from build123d import *

# Parameters (mm, degrees)
F0_W         = 500
F0_H         = 80
F1_DEPTH     = 25
F3_D         = 40
F3_DEPTH     = 25
F3_TIP       = 12.0172123806
F4_D         = 10
F4_DEPTH     = 25
F4_TIP       = 3.0043030951
F2_W         = 38
F2_H         = 28
F5_DEPTH     = 10
F6_T         = 2.5
F6_T3_DEPTH  = 15
F6_T5_DEPTH  = 33
F6_T7_DEPTH  = 29
F6_T9_DEPTH  = 39
F6_T11_DEPTH = 39
F6_T13_DEPTH = 33
F6_T15_DEPTH = 29


# Not quite as in the source:
# - a shell that OpenCascade refuses in one call is made with other operations: the cavity is built on its own and cut out


with BuildPart() as f1:
    # F0 (on Top) → F1 (new body)
    with BuildSketch(Plane.XY):
        Rectangle(F0_W, F0_H)
    extrude(amount=F1_DEPTH)

    # F3
    with Locations(Plane.XY.offset(25)):
        with Locations((0, 0)):
            Hole(F3_D / 2, depth=F3_DEPTH)
            with Locations((0, 0, -(F3_DEPTH + F3_TIP / 2))):  # 118° drill point
                Cone(0, F3_D / 2, F3_TIP, mode=Mode.SUBTRACT)

    # F4
    with Locations(Plane.XY.offset(25)):
        with Locations((-25, 20), (25, 20), (25, -20), (-25, -20)):
            Hole(F4_D / 2, depth=F4_DEPTH)
            with Locations((0, 0, -(F4_DEPTH + F4_TIP / 2))):  # 118° drill point
                Cone(0, F4_D / 2, F4_TIP, mode=Mode.SUBTRACT)

    # F2 (on face) → F5 (cut)
    with BuildSketch(Plane.XY.offset(25)):
        with Locations((-31, -26)):
            Rectangle(F2_W, F2_H)
        with Locations((-31, 26)):
            Rectangle(F2_W, F2_H)
        with Locations((31, 26)):
            Rectangle(F2_W, F2_H)
        with Locations((31, -26)):
            Rectangle(F2_W, F2_H)
    extrude(amount=-F5_DEPTH, mode=Mode.SUBTRACT)

    # F6: shell of thickness 2.5, made by hand


with BuildPart() as f6_core1:
    # F6_t2: copy of F1
    add(f1.part)

    # the walls: a layer under each face that stays
    f6_faces = [f6_core1.faces().sort_by_distance(p)[0] for p in [
        (0, 40, 12.5),
        (-166.6666666667, -26.6666666667, 0),
        (-133, 0, 25),
        (-50, 26, 20),
        (-31, 26, 15),
        (-12, 28, 20),
        (0, 28, 25),
        (12, 28, 20),
        (31, 26, 15),
        (50, 26, 20),
        (133, 0, 25),
        (0, -40, 12.5),
        (-30, -20, 7.5),
        (20, -20, 7.5),
        (-30, 20, 7.5),
        (-20, 0, 12.5),
        (20, 20, 7.5),
        (-33, 12, 20),
        (-33, -12, 20),
        (-50, -26, 20),
        (33, 12, 20),
        (50, -26, 20),
        (33, -12, 20),
        (31, -26, 15),
        (12, -28, 20),
        (0, -28, 25),
        (-12, -28, 20),
        (-31, -26, 15),
    ]]
    thicken(f6_faces, amount=-F6_T, mode=Mode.SUBTRACT)

    # F6_s4 → F6_t3 (cut)
    with BuildSketch(Plane.XY.offset(12.5)):
        Polygon((-49.975, 12.025), (-52.5, 12), (-52.5, 9.5), (-50, 9.5), align=None)
        Polygon((49.975, 12.025), (52.5, 12), (52.5, 9.5), (50, 9.5), align=None)
        Polygon((-49.975, -12.025), (-50, -9.5), (-52.5, -9.5), (-52.5, -12), align=None)
        Polygon((49.975, -12.025), (52.5, -12), (52.5, -9.5), (50, -9.5), align=None)
    extrude(amount=F6_T3_DEPTH, mode=Mode.SUBTRACT)

    # F6_s6 → F6_t5 (cut)
    with BuildSketch(Plane.XZ.offset(-42.5)):
        Polygon((-49.975, 15.025), (-52.5, 15), (-52.5, 12.5), (-50, 12.5), align=None)
        Polygon((49.975, 15.025), (50, 12.5), (52.5, 12.5), (52.5, 15), align=None)
    extrude(amount=F6_T5_DEPTH, mode=Mode.SUBTRACT)

    # F6_s8 → F6_t7 (cut)
    with BuildSketch(Plane.XZ.offset(-42.5)):
        Polygon((-12.025, 15.025), (-12, 12.5), (-9.5, 12.5), (-9.5, 15), align=None)
        Polygon((12.025, 15.025), (9.5, 15), (9.5, 12.5), (12, 12.5), align=None)
    extrude(amount=F6_T7_DEPTH, mode=Mode.SUBTRACT)

    # F6_s10 → F6_t9 (cut)
    with BuildSketch(Plane.YZ.offset(-52.5)):
        Polygon((12.025, 15.025), (12, 12.5), (9.5, 12.5), (9.5, 15), align=None)
        Polygon((-12.025, 15.025), (-9.5, 15), (-9.5, 12.5), (-12, 12.5), align=None)
    extrude(amount=F6_T9_DEPTH, mode=Mode.SUBTRACT)

    # F6_s12 → F6_t11 (cut)
    with BuildSketch(Plane.YZ.offset(13.5)):
        Polygon((12.025, 15.025), (12, 12.5), (9.5, 12.5), (9.5, 15), align=None)
        Polygon((-12.025, 15.025), (-9.5, 15), (-9.5, 12.5), (-12, 12.5), align=None)
    extrude(amount=F6_T11_DEPTH, mode=Mode.SUBTRACT)

    # F6_s14 → F6_t13 (cut)
    with BuildSketch(Plane.XZ.offset(9.5)):
        Polygon((-49.975, 15.025), (-52.5, 15), (-52.5, 12.5), (-50, 12.5), align=None)
        Polygon((49.975, 15.025), (52.5, 15), (52.5, 12.5), (50, 12.5), align=None)
    extrude(amount=F6_T13_DEPTH, mode=Mode.SUBTRACT)

    # F6_s16 → F6_t15 (cut)
    with BuildSketch(Plane.XZ.offset(13.5)):
        Polygon((12.025, 15.025), (12, 12.5), (9.5, 12.5), (9.5, 15), align=None)
        Polygon((-12.025, 15.025), (-9.5, 15), (-9.5, 12.5), (-12, 12.5), align=None)
    extrude(amount=F6_T15_DEPTH, mode=Mode.SUBTRACT)


with BuildPart() as f1_1:
    add(f1.part)

    # what is left inside the walls is the cavity
    f6_cavity = [f6_core1.part.solids().sort_by_distance(p)[0] for p in [
        (-125, 12.5, 2.525),
    ]]
    add(f6_cavity, mode=Mode.SUBTRACT)


solid = f1_1.part
Source: CAD feature listing. Evaluate the final solid. Frame: model axes, mm. A direction names the side the tool comes from. Give positions to 0.01 mm unless a question says otherwise; leave off trailing zeros. Write each loop counter-clockwise with the first axis right and the second up, starting at its lowest first coordinate (ties: lowest second). Pieces come first, ordered by that corner, then holes. Notation, with made-up numbers: M 28.5,-34.75 L 74.5,-34.75 A7 cw 74.5,-27.75 Z; hole C 44,10.25 d10. An arc over 180 degrees is marked long. Return JSON: item names as keys, results as strings. Group by question number.
1) Set-up query: faces 4 (the face through (12, 28, 20)), 5 (the face through (-3, -37.5, 12)), 6 (the face through (-50, 26, 20)). Return all of +Z, -Z, +X, -X, +Y, -Y with unobstructed straight access to the full face (end or side cutting, diameter ignored); none if empty.
2) Cut plane B-B, the plane y = 0. Output: boundary loops of the cut face in (x, z), then the cut area to 3 significant figures.
3) Cut plane A-A, the plane x = 0. Output: boundary loops of the cut face in (y, z).
4) Draft query along Y for faces 1 (the face through (-33, -12, 20)), 2 (the face through (-31, -26, 15)), 3 (the face through (36, 9.5, 18)). Return one class per face: released by +Y, released by -Y, zero draft, split by the parting line, or undercut.
5) Ray query, L1, parallel to Y at x = -25, z = 10.25; L2, parallel to X at y = 28, z = 20.75; L3, parallel to Z at x = -26, y = 1. Return the intervals inside material, ascending.
6) Cut plane C-C, the plane z = 8. Give the number of separate pieces and of enclosed holes in the cut face, then the cut area to 3 significant figures.
7) Cut plane D-D, the plane x = -99. Output: boundary loops of the cut face in (y, z), then the cut area to 3 significant figures.
8) First-contact query: pin 1 Ø5 at (y, z) = (-27.5, 16.5) entering from +X; pin 2 Ø3 at (y, z) = (28, 20.5) entering from -X; pin 3 Ø8 at (y, z) = (5, 16.5) entering from +X. Flat tips, straight axial feed; report the tip coordinate or a pass-through.
Data:
{
 "1": {"face 4": "+Z, +Y, -Y", "face 5": "none", "face 6": "+Z, +Y"},
 "2": {"outline": "M -250,0 L -20,0 L -20,25 L -250,25 L -250,22.5 L -22.5,22.5 L -22.5,2.5 L -250,2.5 Z; M 20,0 L 250,0 L 250,2.5 L 22.5,2.5 L 22.5,22.5 L 250,22.5 L 250,25 L 20,25 Z", "area": "2,400 mm²"},
 "3": {"outline": "M -40,0 L -20,0 L -20,25 L -40,25 Z; M 20,0 L 40,0 L 40,25 L 20,25 Z; hole M -37.5,2.5 L -22.5,2.5 L -22.5,22.5 L -37.5,22.5 Z; hole M 22.5,2.5 L 37.5,2.5 L 37.5,22.5 L 22.5,22.5 Z"},
 "4": {"face 1": "released by -Y", "face 2": "zero draft", "face 3": "undercut"},
 "5": {"L1": "y = -40 to -37.5, -27.5 to -25, -15 to -12.5, 12.5 to 15, 25 to 27.5, 37.5 to 40", "L2": "x = -52.5 to -50, -12 to -9.5, 9.5 to 12, 50 to 52.5", "L3": "z = 0 to 2.5, 22.5 to 25"},
 "6": {"separate pieces": "7", "enclosed holes": "5", "area": "3,230 mm²"},
 "7": {"outline": "M -40,0 L 40,0 L 40,25 L -40,25 Z; hole M -37.5,2.5 L 37.5,2.5 L 37.5,22.5 L -37.5,22.5 Z", "area": "500 mm²"},
 "8": {"pin 1": "stops at x = 52.5", "pin 2": "stops at x = -52.5", "pin 3": "stops at x = 22.48"}
}
